Part model, mm, in its own coordinate system. A direction names the side the tool comes from. Round coordinates to 2 decimals unless told otherwise and drop trailing zeros. Write each loop counter-clockwise with the first axis right and the second up, starting at its lowest first coordinate (ties: lowest second). Pieces come first, ordered by that corner, then holes. Notation, with made-up numbers: (53.25, 36.25) -> (95.25, 36.25) arc R36 ccw to (95.25, 72.25) -> close; hole circle Ø11 at (70, 25). An arc over 180 degrees is marked (long way). Return JSON: item names as keys, results as strings. Group by question number.
```python
from build123d import *

# Parameters (mm, degrees)
F0_W      = 60.96
F0_H      = 104.14
F1_DEPTH  = 10.414
F2_R      = 5.08
F3_R      = 17.78
F3_R_2    = 7.62
F4_DEPTH  = 0.254
F5_R      = 2.54
F6_W      = 45.72
F6_H      = 38.1
F7_DEPTH  = 0.254
F8_R      = 1.763913
F9_DEPTH  = 19.05
F10_W     = 21.063223
F10_H     = 1.628075
F11_DEPTH = 19.05


with BuildPart() as f1:
    # F0 (on Top) → F1 (new body)
    with BuildSketch(Plane.XY):
        with Locations((-7.626853, -3.795236)):
            Rectangle(F0_W, F0_H)
    extrude(amount=F1_DEPTH)

    # F2
    f2_edges = [f1.edges().sort_by_distance(p)[0] for p in [
        (22.853147, 48.274764, 5.207),
        (-38.106853, 48.274764, 5.207),
        (22.853147, -55.865236, 5.207),
        (-38.106853, -55.865236, 5.207),
    ]]
    fillet(f2_edges, radius=F2_R)

    # F3 (on face) → F4 (join)
    with BuildSketch(Plane.XY.offset(10.414)):
        with Locations((-7.626853, -25.385236)):
            Circle(F3_R)
        with Locations((-7.626853, -25.385236)):
            Circle(F3_R_2, mode=Mode.SUBTRACT)
    extrude(amount=F4_DEPTH)

    # F5
    f5_edges = [f1.edges().sort_by_distance(p)[0] for p in [
        (22.853147, -3.795236, 10.414),
        (-38.106853, -3.795236, 0),
    ]]
    fillet(f5_edges, radius=F5_R)

    # F6 (on face) → F7 (cut)
    with BuildSketch(Plane.XY.offset(10.414)):
        with Locations((-7.626853, 19.714694)):
            Rectangle(F6_W, F6_H)
    extrude(amount=-F7_DEPTH, mode=Mode.SUBTRACT)

    # F8 (on face) → F9 (cut)
    with BuildSketch(Plane(origin=(0, 48.274764, 0), x_dir=(-1, 0, 0), z_dir=(0, 1, 0))):
        with Locations((-13.314613, 4.846008)):
            Circle(F8_R)
    extrude(amount=-F9_DEPTH, mode=Mode.SUBTRACT)

    # F10 (on face) → F11 (cut)
    with BuildSketch(Plane.XZ.offset(55.865236)):
        with Locations((-7.410378, 5.054059)):
            Rectangle(F10_W, F10_H)
    extrude(amount=-F11_DEPTH, mode=Mode.SUBTRACT)


solid = f1.part
```
Item 1: Which spindle directions (+Z, -Z, +X, -X, +Y, -Y) get a long thin tool onto all of the face, cutting with end or side? Do faces 1 (the face through (-8, -46, 5.868)), 2 (the face through (-8, -55.865, 4)). Say none if no direction does.
Item 2: Cut at D-D (x = 14). Write the cut outline in (y, z), then the cut area to 3 significant figures.
Item 3: Cut at A-A (y = -1). Write the cut outline in (x, z), then the cut area to 3 significant figures.
Item 4: Flat gauge pins, fed straight in: P1, Ø2, axis at x = 3, y = 35.5, coming from the +Z side; P2, Ø0.5, axis at x = -4, z = 5.5, coming from the -Y side. Where does each tip first touch, or does it go through?
Item 5: Wall check: L1, parallel to Z at x = -14, y = 26; L2, parallel to Z at x = -3, y = -41; L3, parallel to Z at x = -8, y = 39.5. Give the ranges that are in metal, low to high.
Item 6: Cut at C-C (y = -38.5). Write the cut outline in (x, z), then the cut area to 3 significant figures.
Item 7: Two-plate mould, pull along Y, no slides. Class faces 3 (the face through (15.077, 38.883, 4.924)), 4 (the face through (-8, -25, 10.414)), 5 (the face through (-8, 48.275, 5)), 6 (the face through (-7.27, -55.1, 9.69)): released by +Y, released by -Y, zero draft, split by the parting line, or undercut.
Item 8: Cut at B-B (x = 1.5). Write the cut outline in (y, z), then the cut area to 3 significant figures.
Checks:
{
 "1": {"face 1": "-Y", "face 2": "+Z, -Z, +X, -X, -Y"},
 "2": {"outline": "(-55.87, 2.54) arc R2.54 ccw to (-53.33, 0) -> (45.73, 0) arc R2.54 ccw to (48.27, 2.54) -> (48.27, 3.22) -> (29.22, 3.22) -> (29.22, 6.47) -> (48.27, 6.47) -> (48.27, 7.87) arc R2.54 ccw to (45.73, 10.41) -> (38.76, 10.41) -> (38.76, 10.16) -> (0.66, 10.16) -> (0.66, 10.41) -> (-53.33, 10.41) arc R2.54 ccw to (-55.87, 7.87) -> close", "area": "1,010 mm2"},
 "3": {"outline": "(-38.11, 2.54) arc R2.54 ccw to (-35.57, 0) -> (20.31, 0) arc R2.54 ccw to (22.85, 2.54) -> (22.85, 7.87) arc R2.54 ccw to (20.31, 10.41) -> (-35.57, 10.41) arc R2.54 ccw to (-38.11, 7.87) -> close", "area": "629 mm2"},
 "4": {"P1": "stops at z = 10.16", "P2": "stops at y = -36.82"},
 "5": {"L1": "z = 0 to 10.16", "L2": "z = 0 to 4.24, 5.87 to 10.67", "L3": "z = 0 to 10.41"},
 "6": {"outline": "(-38.11, 2.54) arc R2.54 ccw to (-35.57, 0) -> (20.31, 0) arc R2.54 ccw to (22.85, 2.54) -> (22.85, 7.87) arc R2.54 ccw to (20.31, 10.41) -> (4.38, 10.41) -> (4.38, 10.67) -> (-19.63, 10.67) -> (-19.63, 10.41) -> (-35.57, 10.41) arc R2.54 ccw to (-38.11, 7.87) -> close; hole (-17.94, 4.24) -> (3.12, 4.24) -> (3.12, 5.87) -> (-17.94, 5.87) -> close", "area": "601 mm2"},
 "7": {"face 3": "zero draft", "face 4": "undercut", "face 5": "released by +Y", "face 6": "released by -Y"},
 "8": {"outline": "(-55.87, 2.54) arc R2.54 ccw to (-53.33, 0) -> (45.73, 0) arc R2.54 ccw to (48.27, 2.54) -> (48.27, 7.87) arc R2.54 ccw to (45.73, 10.41) -> (38.76, 10.41) -> (38.76, 10.16) -> (0.66, 10.16) -> (0.66, 10.41) -> (-10.13, 10.41) -> (-10.13, 10.67) -> (-40.64, 10.67) -> (-40.64, 10.41) -> (-53.33, 10.41) arc R2.54 ccw to (-55.87, 7.87) -> (-55.87, 5.87) -> (-36.82, 5.87) -> (-36.82, 4.24) -> (-55.87, 4.24) -> close", "area": "1,050 mm2"}
}
